from build123d import *

# Parameters (mm, degrees)
BOSS_EXTRUDE1_DEPTH                               = 10
SKETCH6_W                                         = 13
SKETCH6_H                                         = 23.5
CUT_EXTRUDE1_DEPTH                                = 101.559411442
CSK_FOR_0_FLAT_HEAD_MACHINE_SCREW_100_D           = 1.9304
CSK_FOR_0_FLAT_HEAD_MACHINE_SCREW_100_CSINK_D     = 3.0226
CSK_FOR_0_FLAT_HEAD_MACHINE_SCREW_100_CSINK_ANGLE = 100
SKETCH15_R                                        = 30
BOSS_EXTRUDE2_DEPTH                               = 5


with BuildPart() as part:
    # Sketch4 → Boss-Extrude1 (new body)
    with BuildSketch(Plane.XY):
        with BuildLine():
            Line((39.677308084, 80.316960409), (49.677308084, 80.316960409))
            ThreePointArc((49.677308084, 80.316960409), (56.748375896, 77.388028221), (59.677308084, 70.316960409))
            Line((59.677308084, 70.316960409), (59.677308084, -19.683039591))
            Line((59.677308084, -19.683039591), (29.677308084, -19.683039591))
            Line((29.677308084, -19.683039591), (29.677308084, 70.316960409))
            ThreePointArc((29.677308084, 70.316960409), (32.606240272, 77.388028221), (39.677308084, 80.316960409))
        make_face()
    extrude(amount=BOSS_EXTRUDE1_DEPTH)

    # Sketch6 → Cut-Extrude1 (cut, through all)
    with BuildSketch(Plane.XY.offset(10)):
        with Locations((45.288344904, 57.398882655)):
            Rectangle(SKETCH6_W, SKETCH6_H)
    extrude(amount=-CUT_EXTRUDE1_DEPTH, mode=Mode.SUBTRACT)

    # CSK for #0 Flat Head Machine Screw (100)2 (through all)
    with Locations(Plane.XY.offset(10)):
        with Locations((45.136449354, 72.148882655), (45.136449354, 41.648882655)):
            CounterSinkHole(CSK_FOR_0_FLAT_HEAD_MACHINE_SCREW_100_D / 2, CSK_FOR_0_FLAT_HEAD_MACHINE_SCREW_100_CSINK_D / 2, counter_sink_angle=CSK_FOR_0_FLAT_HEAD_MACHINE_SCREW_100_CSINK_ANGLE)

    # Sketch15 → Boss-Extrude2 (add)
    with BuildSketch(Plane.XZ.offset(19.683039591)):
        with Locations(Location((44.398165665, 5, 0), (0, 0, 270))):
            Circle(SKETCH15_R)
    extrude(amount=BOSS_EXTRUDE2_DEPTH)


solid = part.part
Design review of the part built by this model. Coordinates are the model's own, in mm. A direction names the side the tool comes from. Coordinates: 2 decimals unless noted, no trailing zeros. Order: outer loops, then holes, each group sorted by start corner. A loop starts at its lowest first (then second) coordinate and runs counter-clockwise, first axis right, second up.
Item 1: Take a section at D-D, the plane z = -5.5. Write out the cut boundary in (x, y).
Item 2: For faces 5 (the flat face through (29.677, 25, 5)), 6 (the flat face through (59.677, 26, 5)), 7 (the flat face through (45, 31, 0)), 8 (the flat face through (45, -24.683, 5)), 9 (the flat face through (45, 45.649, 5)), list the 3-axis set-ups (+Z, -Z, +X, -X, +Y, -Y) from which the entire face can be reached by the end or side of a thin tool; tool diameter is ignored.
Item 3: Take a section at A-A, the plane y = 51.5. Write out the cut boundary in (x, z), then the cut area to 3 significant figures.
Item 4: For pin 1 Ø24 at (x, y) = (49.5, 16) entering from -Z; pin 2 Ø5 at (y, z) = (60.5, 3) entering from -X; pin 3 Ø5 at (y, z) = (18.5, 5.5) entering from +X, all flat-tipped, find the tip position at first contact; note any pin that passes through.
Item 5: The part is to be moulded in two halves that separate along Y. For faces 1 (the flat face through (38.788, 57, 5)), 2 (the flat face through (45, 69.149, 5)), 3 (the flat face through (45, 31, 10)), 4 (the cylindrical face through (32.53, 77.31, 4.93)), say which applies: pulls with the +Y half, pulls with the -Y half, needs draft (parallel to the pull), parting line crosses it, or undercut.
Item 6: Take a section at B-B, the plane x = 48.5. Write out the cut boundary in (y, z), then the cut area to 3 significant figures.
Item 7: For line 1 (Y direction, x = 43.5, z = 1); line 2 (Y direction, x = 48.5, z = -4); line 3 (X direction, y = 69, z = 4.5), list the stretches that pass through material, from the lowest coordinate up.
Item 8: Take a section at C-C, the plane z = 2.5. Write out the cut boundary in (x, y).
The answers:
1. outline: (16.3, -24.68) - (72.5, -24.68) - (72.5, -19.68) - (16.3, -19.68) - close
2. face 5: +Z, -Z, -X, +Y
2. face 6: +Z, -Z, +X, +Y
2. face 7: -Z, +X, -X, +Y
2. face 8: +Z, -Z, +X, -X, -Y
2. face 9: +Z, -Z
3. outline: (29.68, 0) - (38.79, 0) - (38.79, 10) - (29.68, 10) - close; (51.79, 0) - (59.68, 0) - (59.68, 10) - (51.79, 10) - close
3. area: 170 mm2
4. pin 1: stops at z = 0
4. pin 2: stops at x = 29.68
4. pin 3: stops at x = 59.68
5. face 1: undercut
5. face 2: undercut
5. face 3: needs draft
5. face 4: pulls with the +Y half
6. outline: (-24.68, -24.72) - (-19.68, -24.72) - (-19.68, 0) - (45.65, 0) - (45.65, 10) - (-19.68, 10) - (-19.68, 34.72) - (-24.68, 34.72) - close; (69.15, 0) - (80.32, 0) - (80.32, 10) - (69.15, 10) - close
6. area: 1,060 mm2
7. line 1: y = -24.68 to 45.65, 69.15 to 80.32
7. line 2: y = -24.68 to -19.68
7. line 3: x = 29.68 to 38.79, 51.79 to 59.68
8. outline: (14.5, -24.68) - (74.29, -24.68) - (74.29, -19.68) - (59.68, -19.68) - (59.68, 70.32) arc R10 ccw to (49.68, 80.32) - (39.68, 80.32) arc R10 ccw to (29.68, 70.32) - (29.68, -19.68) - (14.5, -19.68) - close; hole (38.79, 45.65) - (51.79, 45.65) - (51.79, 69.15) - (38.79, 69.15) - close; hole circle Ø1.93 at (45.14, 41.65); hole circle Ø1.93 at (45.14, 72.15)
